For this review, take the finished solid that the model builds, in its own axes (mm). A direction names the side the tool comes from. Round coordinates to 2 decimals unless told otherwise and drop trailing zeros. Write each loop counter-clockwise with the first axis right and the second up, starting at its lowest first coordinate (ties: lowest second). Pieces come first, ordered by that corner, then holes.
from build123d import *

# Parameters (mm, degrees)
BOSS_EXTRUDE1_DEPTH = 30
BOSS_EXTRUDE2_DEPTH = 5
CUT_EXTRUDE1_START  = -69
CUT_EXTRUDE1_DEPTH  = 69
BOSS_EXTRUDE3_START = 5
BOSS_EXTRUDE3_DEPTH = 5
SKETCH7_R           = 2.25
CUT_EXTRUDE3_DEPTH  = 12.5
SKETCH8_R           = 2.25
CUT_EXTRUDE4_DEPTH  = 12.5


with BuildPart() as part:
    # Sketch1 → Boss-Extrude1 (new body)
    with BuildSketch(Plane.XY):
        Polygon((-27.5, -14.382195086), (27.5, -14.382195086), (22.5, -19.382195086), (45, -19.382195086), (45, -4.382195086), (35, -4.382195086), (35, 5.617804914), (-35, 5.617804914), (-35, -4.382195086), (-45, -4.382195086), (-45, -19.382195086), (-22.5, -19.382195086), align=None)
    extrude(amount=-BOSS_EXTRUDE1_DEPTH)

    # Sketch2 → Boss-Extrude2 (add)
    with BuildSketch(Plane.XY):
        with BuildLine():
            Line((-10, 5.617804914), (10, 5.617804914))
            ThreePointArc((10, 5.617804914), (17.5, -1.882195086), (25, 5.617804914))
            Line((25, 5.617804914), (30, 5.617804914))
            ThreePointArc((30, 5.617804914), (26.338834765, -3.221029851), (17.5, -6.882195086))
            Line((17.5, -6.882195086), (7.5, -6.882195086))
            Line((7.5, -6.882195086), (7.5, -14.382195086))
            Line((7.5, -14.382195086), (-7.5, -14.382195086))
            Line((-7.5, -14.382195086), (-7.5, -6.882195086))
            Line((-7.5, -6.882195086), (-17.5, -6.882195086))
            ThreePointArc((-17.5, -6.882195086), (-26.338834765, -3.221029851), (-30, 5.617804914))
            Line((-30, 5.617804914), (-25, 5.617804914))
            ThreePointArc((-25, 5.617804914), (-17.5, -1.882195086), (-10, 5.617804914))
        make_face()
    extrude(amount=BOSS_EXTRUDE2_DEPTH)

    # Sketch3 → Cut-Extrude1 (cut)
    with BuildSketch(Plane.XY.offset(5).offset(CUT_EXTRUDE1_START)):
        with BuildLine():
            Line((-25, 5.617804914), (-10, 5.617804914))
            ThreePointArc((-10, 5.617804914), (-17.5, -1.882195086), (-25, 5.617804914))
        make_face()
        with BuildLine():
            Line((10, 5.617804914), (25, 5.617804914))
            ThreePointArc((25, 5.617804914), (17.5, -1.882195086), (10, 5.617804914))
        make_face()
    extrude(amount=CUT_EXTRUDE1_DEPTH, mode=Mode.SUBTRACT)

    # Sketch4 → Boss-Extrude3 (add)
    with BuildSketch(Plane(origin=(0, 0, -30), x_dir=(-1, 0, 0), z_dir=(0, 0, -1)).offset(BOSS_EXTRUDE3_START)):
        with BuildLine():
            Line((-17.5, -6.882195086), (-7.5, -6.882195086))
            Line((-7.5, -6.882195086), (-7.5, -14.382195086))
            Line((-7.5, -14.382195086), (7.5, -14.382195086))
            Line((7.5, -14.382195086), (7.5, -6.882195086))
            Line((7.5, -6.882195086), (17.5, -6.882195086))
            ThreePointArc((17.5, -6.882195086), (26.338834765, -3.221029851), (30, 5.617804914))
            Line((30, 5.617804914), (25, 5.617804914))
            ThreePointArc((25, 5.617804914), (17.5, -1.882195086), (10, 5.617804914))
            Line((10, 5.617804914), (-10, 5.617804914))
            ThreePointArc((-10, 5.617804914), (-17.5, -1.882195086), (-25, 5.617804914))
            Line((-25, 5.617804914), (-30, 5.617804914))
            ThreePointArc((-30, 5.617804914), (-26.338834765, -3.221029851), (-17.5, -6.882195086))
        make_face()
    extrude(amount=-BOSS_EXTRUDE3_DEPTH)

    # Sketch7 → Cut-Extrude3 (cut)
    with BuildSketch(Plane(origin=(0, 5.617804914, 0), x_dir=(1, 0, 0), z_dir=(0, 1, 0))):
        with Locations(Location((0, 30, 0), (0, 0, 270))):
            Circle(SKETCH7_R)
        with Locations(Location((0, 0, 0), (0, 0, 270))):
            Circle(SKETCH7_R)
    extrude(amount=-CUT_EXTRUDE3_DEPTH, mode=Mode.SUBTRACT)

    # Sketch8 → Cut-Extrude4 (cut)
    with BuildSketch(Plane(origin=(0, 5.617804914, 0), x_dir=(1, 0, 0), z_dir=(0, 1, 0))):
        with Locations(Location((30, 22.419418388, 0), (0, 0, 270))):
            Circle(SKETCH8_R)
        with Locations(Location((30, 6.707708861, 0), (0, 0, 270))):
            Circle(SKETCH8_R)
        with Locations(Location((-30, 6.707708861, 0), (0, 0, 90))):
            Circle(SKETCH8_R)
        with Locations(Location((-30, 22.419418388, 0), (0, 0, 90))):
            Circle(SKETCH8_R)
    extrude(amount=-CUT_EXTRUDE4_DEPTH, mode=Mode.SUBTRACT)


solid = part.part
(1) For faces 4 (the face through (-26.24, -3.32, 2.46)), 5 (the face through (0.676, -0.545, 2.146)), 6 (the face through (35, 1, -15)), 7 (the face through (13, -6.882, 2)), list the 3-axis set-ups (+Z, -Z, +X, -X, +Y, -Y) from which the entire face can be reached by the end or side of a thin tool; tool diameter is ignored.
Geometry check:
face 4: +Z, -X, -Y
face 5: +Y
face 6: +Z, -Z, +X, +Y
face 7: +Z, +X, -Y
(2) We need section A-A, the plane y = 1. State how many separate pieces and enclosed holes the cut face has, and give its area (3 significant figures).
Geometry check:
separate pieces: 3
enclosed holes: 6
area: 1,640 mm2
(3) For line 1 along Z through (x, y) = (-30, -2); line 2 along X through (y, z) = (-2.5, -8.5); line 3 along Y through (x, z) = (-41, -9), list the stretches that pass through material, from the lowest coordinate up.
Geometry check:
line 1: z = -30 to -24.67, -20.17 to -8.96, -4.46 to 0
line 2: x = -35 to -31.36, -28.64 to 28.64, 31.36 to 35
line 3: y = -19.38 to -4.38
(4) Mouldability with a two-part tool opening along X and no side actions: class faces 1 (the face through (-12, -6.882, -33)), 2 (the face through (26.44, -3.12, 2.46)), 3 (the face through (0, -14.382, -15)) as pulls with the +X half, pulls with the -X half, needs draft (parallel to the pull), parting line crosses it, or undercut.
Geometry check:
face 1: needs draft
face 2: pulls with the +X half
face 3: undercut
(5) We need section B-B, the plane x = 0. Give the boundary of the cut face in (y, z).
Geometry check:
outline: (-14.38, -35) - (5.62, -35) - (5.62, -32.25) - (-6.88, -32.25) - (-6.88, -27.75) - (5.62, -27.75) - (5.62, -2.25) - (-6.88, -2.25) - (-6.88, 2.25) - (5.62, 2.25) - (5.62, 5) - (-14.38, 5) - close
(6) We need section D-D, the plane x = 14. Give the boundary of the cut face in (y, z), and give its area (3 significant figures).
Geometry check:
outline: (-14.38, -30) - (-6.88, -30) - (-6.88, -35) - (-1.02, -35) - (-1.02, 5) - (-6.88, 5) - (-6.88, 0) - (-14.38, 0) - close
area: 460 mm2
(7) For pin 1 Ø1.5 at (y, z) = (-11.5, 2.5) entering from +X; pin 2 Ø7.5 at (x, y) = (-34, -8) entering from +Z; pin 3 Ø3 at (x, z) = (39, -14.5) entering from +Y, all flat-tipped, find the tip position at first contact; note any pin that passes through.
Geometry check:
pin 1: stops at x = 7.5
pin 2: stops at z = 0
pin 3: stops at y = -4.38
(8) We need section C-C, the plane x = -13. Give the boundary of the cut face in (y, z).
Geometry check:
outline: (-14.38, -30) - (-6.88, -30) - (-6.88, -35) - (-0.38, -35) - (-0.38, 5) - (-6.88, 5) - (-6.88, 0) - (-14.38, 0) - close
